For this review, take the finished solid that the model builds, in its own axes (mm). A direction names the side the tool comes from. Round coordinates to 2 decimals unless told otherwise and drop trailing zeros. Write each loop counter-clockwise with the first axis right and the second up, starting at its lowest first coordinate (ties: lowest second). Pieces come first, ordered by that corner, then holes. Notation, with made-up numbers: M 51,75.5 L 82,75.5 A10 cw 82,86.5 Z; hole C 19.5,-37 d6. An arc over 180 degrees is marked long. One line per question, with ' | ' between items.
```python
from build123d import *

# Parameters (mm, degrees)
F0_W     = 34.57
F0_H     = 9
F0_H_2   = 8.8497422612
F1_DEPTH = 3
F3_D     = 6.6
F5_DEPTH = 25


with BuildPart() as f1:
    # F0 (on Top) → F1 (new body)
    with BuildSketch(Plane.XY):
        with Locations((-2.915, 8.9248711306)):
            Rectangle(F0_W, F0_H)
        with Locations((-2.915, 0)):
            Rectangle(F0_W, F0_H_2)
        Polygon((-15.1, 2.4248711306), (-13, 1.2124355653), (-13, -1.2124355653), (-15.1, -2.4248711306), (-17.2, -1.2124355653), (-17.2, 1.2124355653), align=None, mode=Mode.SUBTRACT)
        Polygon((-9.4, 1.8475208614), (-7.8, 0.9237604307), (-7.8, -0.9237604307), (-9.4, -1.8475208614), (-11, -0.9237604307), (-11, 0.9237604307), align=None, mode=Mode.SUBTRACT)
        Polygon((-4.45, 1.5588457268), (-3.1, 0.7794228634), (-3.1, -0.7794228634), (-4.45, -1.5588457268), (-5.8, -0.7794228634), (-5.8, 0.7794228634), align=None, mode=Mode.SUBTRACT)
        Polygon((0, 1.2701705922), (1.1, 0.6350852961), (1.1, -0.6350852961), (0, -1.2701705922), (-1.1, -0.6350852961), (-1.1, 0.6350852961), align=None, mode=Mode.SUBTRACT)
        Polygon((3.95, 0.9814954576), (4.8, 0.4907477288), (4.8, -0.4907477288), (3.95, -0.9814954576), (3.1, -0.4907477288), (3.1, 0.4907477288), align=None, mode=Mode.SUBTRACT)
        Polygon((7.54, 0.8544783984), (8.28, 0.4272391992), (8.28, -0.4272391992), (7.54, -0.8544783984), (6.8, -0.4272391992), (6.8, 0.4272391992), align=None, mode=Mode.SUBTRACT)
        Polygon((10.825, 0.6293117934), (11.37, 0.3146558967), (11.37, -0.3146558967), (10.825, -0.6293117934), (10.28, -0.3146558967), (10.28, 0.3146558967), align=None, mode=Mode.SUBTRACT)
    extrude(amount=F1_DEPTH)

    # F3 (through all)
    with Locations(Plane.XY.offset(3)):
        with Locations((-15.2, 9.3164853752), (9.37, 9.3164853752)):
            Hole(F3_D / 2)

    # F4 (on face) → F5 (cut)
    with BuildSketch(Plane.XY.offset(3)):
        with BuildLine():
            Line((9.3698995221, 12.6164853736), (-15.1298372011, 12.6157394093))
            ThreePointArc((-15.1298372011, 12.6157394093), (-12.8418717978, 11.6249981826), (-11.9, 9.3164853752))
            ThreePointArc((-11.9, 9.3164853752), (-12.866547622, 6.9830329973), (-15.1999999998, 6.0164853752))
            Line((-15.1999999998, 6.0164853752), (9.3698995221, 6.0164853767))
            ThreePointArc((9.3698995221, 6.0164853767), (6.07, 9.3164853752), (9.3698995221, 12.6164853736))
        make_face()
    extrude(amount=-F5_DEPTH, mode=Mode.SUBTRACT)


solid = f1.part
```
Item 1: Take a section at C-C (z = 1). State how many separate pieces and enclosed holes the cut face has, then the cut area to 3 significant figures.
Results:
separate pieces: 1 | enclosed holes: 8 | area: 381 mm2
Item 2: Take a section at A-A (y = 12.25). Write out the cut boundary in (x, z).
Results:
outline: M -20.2,0 L -16.71,0 L -16.71,3 L -20.2,3 Z; M 10.88,0 L 14.37,0 L 14.37,3 L 10.88,3 Z
Item 3: Machinability: for faces 1 (the face through (-5.12, -1.17, 1.48)), 2 (the face through (14.37, 4, 1)), which of the approach directions +Z, -Z, +X, -X, +Y, -Y give a long, thin tool a straight path to every point of the face, cutting with its end or side? Answer none if there is none.
Results:
face 1: +Z, -Z | face 2: +Z, -Z, +X, +Y, -Y
Item 4: To check wall thickness, follow line 1 along Y through (x, z) = (-10.5, 1.8); line 2 along X through (y, z) = (9.25, 1.6); line 3 along Y through (x, z) = (-9.5, 2.75). State the ranges of each line that lie inside material, in increasing order. Write a range as from..to.
Results:
line 1: -4.42..-1.21, 1.21..6.02, 12.62..13.42 | line 2: -20.2..-18.5, 12.67..14.37 | line 3: -4.42..-1.79, 1.79..6.02, 12.62..13.42
Item 5: Take a section at B-B (x = 2). Write out the cut boundary in (y, z).
Results:
outline: M -4.42,0 L 6.02,0 L 6.02,3 L -4.42,3 Z; M 12.62,0 L 13.42,0 L 13.42,3 L 12.62,3 Z
Item 6: Mouldability with a two-part tool opening along Y and no side actions: class faces 3 (the face through (-3, 3, 3)), 4 (the face through (-3, -4.425, 1)), 5 (the face through (-0.558, 0.948, 1.479)), 6 (the face through (-0.54, -0.96, 1.48)) as +Y half, -Y half, draft (parallel to the pull), parting line (faces both ways), or undercut.
Results:
face 3: draft | face 4: -Y half | face 5: undercut | face 6: undercut
